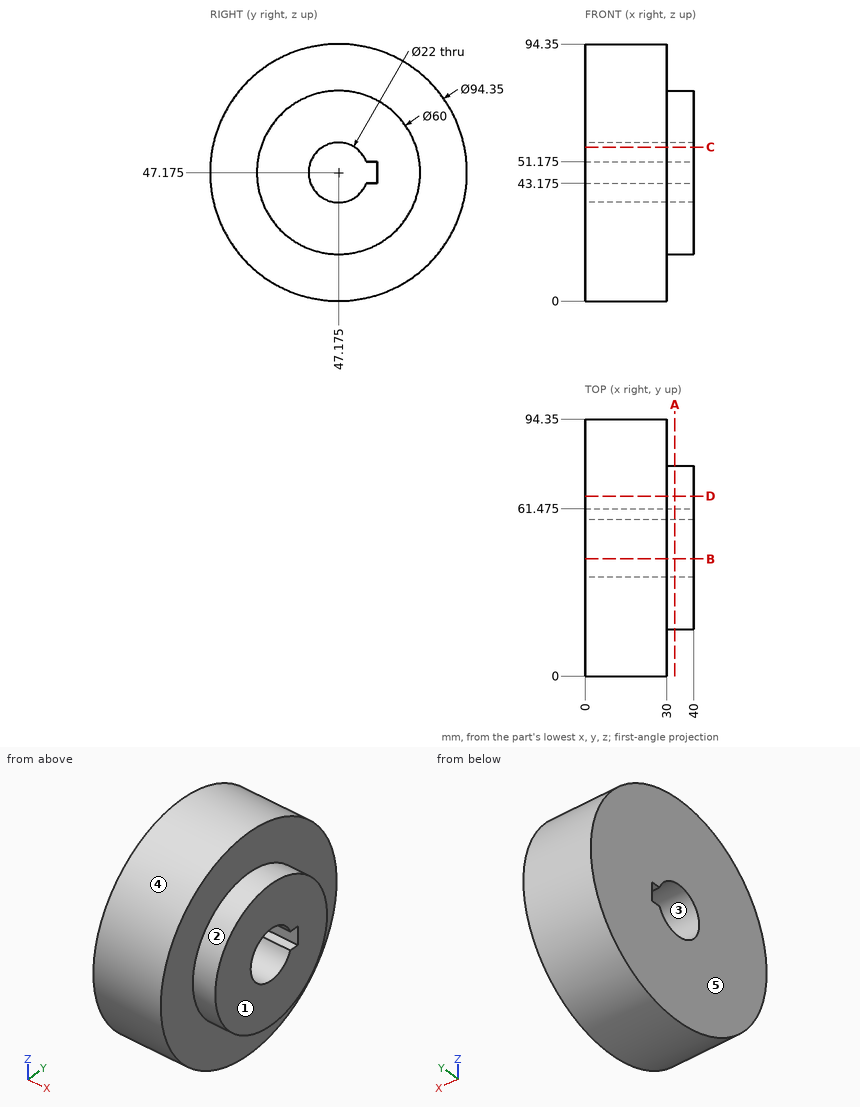
Could you check a few things on this drawing? It's one solid part, dimensions in mm from its lowest x, y, z. A direction names the side the tool comes from. Give positions to 0.01 mm unless a question says otherwise; leave off trailing zeros. Write each loop counter-clockwise with the first axis right and the second up, starting at its lowest first coordinate (ties: lowest second). Pieces come first, ordered by that corner, then holes. Notation, with made-up numbers: (-19, -2.75) -> (15, -2.75) arc R32 ccw to (15, 24.25) -> close; hole circle Ø4 at (38.25, 51). An arc over 180 degrees is marked (long way). Write each question's results on one line, items separated by ' | '.
1. Will these pins go through, and if not, where does the flat tip stop? pin 1 Ø6 at (x, y) = (19.5, 74.5) entering from -Z (3 decimals); pin 2 Ø10 at (x, z) = (29, 41) entering from -Y; pin 3 Ø3 at (x, y) = (17, 59) entering from +Z.
Check sheet entries:
pin 1: stops at z = 6.755 | pin 2: stops at y = 0.01 | pin 3: stops at z = 93.21
2. If we mould it in two halves opening along Z, with no side actions, what happens to the marked faces 3, 4 and 5? For each: released by +Z, released by -Z, zero draft, split by the parting line, or undercut.
Check sheet entries:
face 3: undercut | face 4: split by the parting line | face 5: zero draft
3. I want a section at A-A, the plane x = 33. Write out the boundary of the cut face in (y, z) (3 decimals).
Check sheet entries:
outline: circle Ø60 at (47.175, 47.175); hole (57.422, 43.175) -> (61.475, 43.175) -> (61.475, 51.175) -> (57.422, 51.175) arc R11 ccw (long way) to start
4. On a 3-axis mill with a long thin cutter (end or side, diameter ignored), from which of +Z, -Z, +X, -X, +Y, -Y can I reach the whole of each face in a straight line? I mean the marked faces 1 and 2. Say none if no direction works.
Check sheet entries:
face 1: +Z, -Z, +X, +Y, -Y | face 2: +X
5. I want a section at C-C, the plane z = 56.5. Write out the boundary of the cut face in (x, y), then the cut area to 3 significant figures.
Check sheet entries:
outline: (0, 0.93) -> (30, 0.93) -> (30, 18.66) -> (40, 18.66) -> (40, 41.34) -> (0, 41.34) -> close; (0, 53.01) -> (40, 53.01) -> (40, 75.69) -> (30, 75.69) -> (30, 93.42) -> (0, 93.42) -> close | area: 2,880 mm²
6. I want a section at D-D, the plane y = 66. Write out the boundary of the cut face in (x, z), then the cut area to 3 significant figures.
Check sheet entries:
outline: (0, 3.92) -> (30, 3.92) -> (30, 23.82) -> (40, 23.82) -> (40, 70.53) -> (30, 70.53) -> (30, 90.43) -> (0, 90.43) -> close | area: 3,060 mm²
7. I need wall thicknesses on L1, parallel to Y at x = 28, z = 48 (3 decimals); L2, parallel to X at y = 67, z = 73; L3, parallel to Z at x = 38, y = 57. Which ranges of each line are inside material? Lowest first, please.
Check sheet entries:
L1: y = 0.007 to 36.206, 61.475 to 94.343 | L2: x = 0 to 30 | L3: z = 18.83 to 42.23, 52.12 to 75.52
8. I want a section at B-B, the plane y = 43. Write out the boundary of the cut face in (x, z), then the cut area to 3 significant figures.
Check sheet entries:
outline: (0, 0.19) -> (30, 0.19) -> (30, 17.47) -> (40, 17.47) -> (40, 37) -> (0, 37) -> close; (0, 57.35) -> (40, 57.35) -> (40, 76.88) -> (30, 76.88) -> (30, 94.16) -> (0, 94.16) -> close | area: 2,600 mm²
